Part model, mm, in its own coordinate system. A direction names the side the tool comes from. Round coordinates to 2 decimals unless told otherwise and drop trailing zeros. Loops run counter-clockwise (first coordinate to the right, second up) from the corner with the lowest first, then second, coordinate; pieces in that order, holes last. Notation, with made-up numbers: M 68.5,-22.75 L 111.5,-22.75 A16 ccw 111.5,-10.75 Z; hole C -9.75,32.25 d5. An arc over 180 degrees is marked long. Answer as CSV lines item,"result". Start each with the question number.
Item 1: Mould opens along X. For faces 1 (the cylindrical face through (-24, 51, 0)), 2 (the flat face through (-3, 22, -21)), 3 (the flat face through (-26, 19, 0)) say: pulls with the +X half, pulls with the -X half, needs draft (parallel to the pull), parting line crosses it, or undercut.
Item 2: Band-saw the part on B-B (z = -14.5). Count the separate pieces of the cut face and the enclosed holes in it, and give its area (3 significant figures).
Item 3: Band-saw the part on D-D (y = 47). Give the cut face in (x, z), and give its area (3 significant figures).
Item 4: Drop flat-ended pins along their axis: pin 1 Ø1.2 at (x, z) = (-25.5, 7.5) entering from -Y; pin 2 Ø6 at (x, z) = (-5, 11.5) entering from -Y. Give the stop position or say it passes through.
Item 5: Which spindle directions (+Z, -Z, +X, -X, +Y, -Y) get a long thin tool onto all of the face, cutting with end or side? Do faces 4 (the flat face through (-3, 37, -21)), 5 (the flat face through (-26, 58, 0)), 6 (the flat face through (-28, 53, 0)), 7 (the flat face through (-3, 55, 21)). Say none if no direction does.
Item 6: Wall check: line 1 (Z direction, x = 16.5, y = 57); line 2 (X direction, y = 18, z = 0); line 3 (Z direction, x = -16.5, y = 8.5). Give the ranges that are in metal, low to high.
Item 7: Band-saw the part on A-A (y = 56). Give the cut face in (x, z).
```python
from build123d import *

# Parameters (mm, degrees)
BOSS_EXTRUDE1_DEPTH     = 62
SKETCH2_R               = 18
BOSS_EXTRUDE2_DEPTH     = 2
SKETCH3_R               = 16
CUT_EXTRUDE1_DEPTH      = 65
CUT_EXTRUDE2_DEPTH      = 2
SKETCH6_R               = 3.5
CUT_EXTRUDE3_DEPTH      = 65
SKETCH7_W               = 48
SKETCH7_H               = 3
LPATTERN1_COUNT         = 9
LPATTERN1_PITCH         = 6
MIRROR1_COPY_1_SKETCH_W = 48
MIRROR1_COPY_1_SKETCH_H = 3
MIRROR1_COPY_2_SKETCH_W = 48
MIRROR1_COPY_2_SKETCH_H = 3
MIRROR1_COPY_3_SKETCH_W = 48
MIRROR1_COPY_3_SKETCH_H = 3
MIRROR1_COPY_4_SKETCH_W = 48
MIRROR1_COPY_4_SKETCH_H = 3
MIRROR1_COPY_5_SKETCH_W = 48
MIRROR1_COPY_5_SKETCH_H = 3
MIRROR1_COPY_6_SKETCH_W = 48
MIRROR1_COPY_6_SKETCH_H = 3
MIRROR1_COPY_7_SKETCH_W = 48
MIRROR1_COPY_7_SKETCH_H = 3
MIRROR1_COPY_8_SKETCH_W = 48
MIRROR1_COPY_8_SKETCH_H = 3
SKETCH9_W               = 48
SKETCH9_H               = 3
LPATTERN2_COUNT         = 9
LPATTERN2_PITCH         = 6


with BuildPart() as part:
    # Sketch1 → Boss-Extrude1 (new body)
    with BuildSketch(Plane(origin=(0, 0, 0), x_dir=(1, 0, 0), z_dir=(0, 1, 0))):
        with BuildLine():
            Line((-24, 22.5), (18, 22.5))
            ThreePointArc((18, 22.5), (20.828427125, 21.328427125), (22, 18.5))
            Line((22, 18.5), (22, -18.5))
            ThreePointArc((22, -18.5), (20.828427125, -21.328427125), (18, -22.5))
            Line((18, -22.5), (-24, -22.5))
            ThreePointArc((-24, -22.5), (-26.828427125, -21.328427125), (-28, -18.5))
            Line((-28, -18.5), (-28, 18.5))
            ThreePointArc((-28, 18.5), (-26.828427125, 21.328427125), (-24, 22.5))
        make_face()
    extrude(amount=BOSS_EXTRUDE1_DEPTH)

    # Sketch2 → Boss-Extrude2 (add)
    with BuildSketch(Plane.XZ):
        Circle(SKETCH2_R)
    extrude(amount=BOSS_EXTRUDE2_DEPTH)

    # Sketch3 → Cut-Extrude1 (cut, through all)
    with BuildSketch(Plane.XZ.offset(2)):
        Circle(SKETCH3_R)
    extrude(amount=-CUT_EXTRUDE1_DEPTH, mode=Mode.SUBTRACT)

    # Sketch5 → Cut-Extrude2 (cut)
    with BuildSketch(Plane(origin=(0, 62, 0), x_dir=(1, 0, 0), z_dir=(0, 1, 0))):
        with BuildLine():
            Line((-22.61, 2), (-11.427293838, 2))
            Line((-11.427293838, 2), (-11.427293838, -2))
            Line((-11.427293838, -2), (-22.61, -2))
            ThreePointArc((-22.61, -2), (-24.61, 0), (-22.61, 2))
        make_face()
    extrude(amount=-CUT_EXTRUDE2_DEPTH, mode=Mode.SUBTRACT)

    # Sketch6 → Cut-Extrude3 (cut, through all)
    with BuildSketch(Plane(origin=(0, 62, 0), x_dir=(1, 0, 0), z_dir=(0, 1, 0))):
        with Locations((16.263455967, 16.263455967)):
            Circle(SKETCH6_R)
        with Locations((16.263455967, -16.263455967)):
            Circle(SKETCH6_R)
        with Locations((-16.263455967, -16.263455967)):
            Circle(SKETCH6_R)
        with Locations((-16.263455967, 16.263455967)):
            Circle(SKETCH6_R)
    extrude(amount=-CUT_EXTRUDE3_DEPTH, mode=Mode.SUBTRACT)

    # Sketch7 → Cut-Revolve1 (revolve, cut)
    with BuildSketch(Plane(origin=(-3, 0, 0), x_dir=(0, 0, -1), z_dir=(1, 0, 0))):
        with Locations((-42.5, 56.5)):
            Rectangle(SKETCH7_W, SKETCH7_H)
    cut_revolve1 = revolve(axis=Axis((-3, 58, 66.5), (0, -1, 0)), mode=Mode.SUBTRACT)

    # LPattern1: Cut-Revolve1 ×9
    with Locations(*[(0, -i * LPATTERN1_PITCH, 0) for i in range(1, LPATTERN1_COUNT)]):
        add(cut_revolve1, mode=Mode.SUBTRACT)

    # Mirror1: Cut-Revolve1 across plane
    add(cut_revolve1.mirror(Plane.XY), mode=Mode.SUBTRACT)

    # Mirror1 copy 1 sketch → Mirror1 copy 1 (revolve, cut)
    with BuildSketch(Plane(origin=(-3, -6, 0), x_dir=(0, 0, 1), z_dir=(1, 0, 0))):
        with Locations((-42.5, -56.5)):
            Rectangle(MIRROR1_COPY_1_SKETCH_W, MIRROR1_COPY_1_SKETCH_H)
    revolve(axis=Axis((-3, 52, -66.5), (0, 1, 0)), mode=Mode.SUBTRACT)

    # Mirror1 copy 2 sketch → Mirror1 copy 2 (revolve, cut)
    with BuildSketch(Plane(origin=(-3, -12, 0), x_dir=(0, 0, 1), z_dir=(1, 0, 0))):
        with Locations((-42.5, -56.5)):
            Rectangle(MIRROR1_COPY_2_SKETCH_W, MIRROR1_COPY_2_SKETCH_H)
    revolve(axis=Axis((-3, 46, -66.5), (0, 1, 0)), mode=Mode.SUBTRACT)

    # Mirror1 copy 3 sketch → Mirror1 copy 3 (revolve, cut)
    with BuildSketch(Plane(origin=(-3, -18, 0), x_dir=(0, 0, 1), z_dir=(1, 0, 0))):
        with Locations((-42.5, -56.5)):
            Rectangle(MIRROR1_COPY_3_SKETCH_W, MIRROR1_COPY_3_SKETCH_H)
    revolve(axis=Axis((-3, 40, -66.5), (0, 1, 0)), mode=Mode.SUBTRACT)

    # Mirror1 copy 4 sketch → Mirror1 copy 4 (revolve, cut)
    with BuildSketch(Plane(origin=(-3, -24, 0), x_dir=(0, 0, 1), z_dir=(1, 0, 0))):
        with Locations((-42.5, -56.5)):
            Rectangle(MIRROR1_COPY_4_SKETCH_W, MIRROR1_COPY_4_SKETCH_H)
    revolve(axis=Axis((-3, 34, -66.5), (0, 1, 0)), mode=Mode.SUBTRACT)

    # Mirror1 copy 5 sketch → Mirror1 copy 5 (revolve, cut)
    with BuildSketch(Plane(origin=(-3, -30, 0), x_dir=(0, 0, 1), z_dir=(1, 0, 0))):
        with Locations((-42.5, -56.5)):
            Rectangle(MIRROR1_COPY_5_SKETCH_W, MIRROR1_COPY_5_SKETCH_H)
    revolve(axis=Axis((-3, 28, -66.5), (0, 1, 0)), mode=Mode.SUBTRACT)

    # Mirror1 copy 6 sketch → Mirror1 copy 6 (revolve, cut)
    with BuildSketch(Plane(origin=(-3, -36, 0), x_dir=(0, 0, 1), z_dir=(1, 0, 0))):
        with Locations((-42.5, -56.5)):
            Rectangle(MIRROR1_COPY_6_SKETCH_W, MIRROR1_COPY_6_SKETCH_H)
    revolve(axis=Axis((-3, 22, -66.5), (0, 1, 0)), mode=Mode.SUBTRACT)

    # Mirror1 copy 7 sketch → Mirror1 copy 7 (revolve, cut)
    with BuildSketch(Plane(origin=(-3, -42, 0), x_dir=(0, 0, 1), z_dir=(1, 0, 0))):
        with Locations((-42.5, -56.5)):
            Rectangle(MIRROR1_COPY_7_SKETCH_W, MIRROR1_COPY_7_SKETCH_H)
    revolve(axis=Axis((-3, 16, -66.5), (0, 1, 0)), mode=Mode.SUBTRACT)

    # Mirror1 copy 8 sketch → Mirror1 copy 8 (revolve, cut)
    with BuildSketch(Plane(origin=(-3, -48, 0), x_dir=(0, 0, 1), z_dir=(1, 0, 0))):
        with Locations((-42.5, -56.5)):
            Rectangle(MIRROR1_COPY_8_SKETCH_W, MIRROR1_COPY_8_SKETCH_H)
    revolve(axis=Axis((-3, 10, -66.5), (0, 1, 0)), mode=Mode.SUBTRACT)

    # Sketch9 → Cut-Revolve3 (revolve, cut)
    with BuildSketch(Plane.XY):
        with Locations((-48, 56.5)):
            Rectangle(SKETCH9_W, SKETCH9_H)
    cut_revolve3 = revolve(axis=Axis((-72, 58, 0), (0, -1, 0)), mode=Mode.SUBTRACT)

    # LPattern2: Cut-Revolve3 ×9
    with Locations(*[(0, -i * LPATTERN2_PITCH, 0) for i in range(1, LPATTERN2_COUNT)]):
        add(cut_revolve3, mode=Mode.SUBTRACT)


solid = part.part
```
Answer block:
1,face 1,"pulls with the -X half"
1,face 2,"undercut"
1,face 3,"needs draft"
2,separate pieces,"4"
2,enclosed holes,"0"
2,area,"1,480 mm^2"
3,outline,"M -28,-18.5 A4 ccw -24,-22.5 L 18,-22.5 A4 ccw 22,-18.5 L 22,18.5 A4 ccw 18,22.5 L -24,22.5 A4 ccw -28,18.5 Z; hole C -16.26,-16.26 d7; hole C -16.26,16.26 d7; hole C 0,0 d32; hole C 16.26,-16.26 d7; hole C 16.26,16.26 d7"
3,area,"1,280 mm^2"
4,pin 1,"stops at y = 0"
4,pin 2,"passes through"
5,face 4,"-Z"
5,face 5,"-X"
5,face 6,"+Z, -Z, -X, +Y, -Y"
5,face 7,"+Z"
6,line 1,"z = -22.5 to -19.76, -12.77 to 12.77, 19.76 to 22.5"
6,line 2,"x = -28 to -16, 16 to 22"
6,line 3,"z = -20.44 to -19.76, -12.77 to 12.77, 19.76 to 20.44"
7,outline,"M -27.96,-19.08 A4 ccw -24,-22.5 L -22.18,-22.5 A48 cw 16.18,-22.5 L 18,-22.5 A4 ccw 22,-18.5 L 22,18.5 A4 ccw 18,22.5 L 16.18,22.5 A48 cw -22.18,22.5 L -24,22.5 A4 ccw -27.96,19.08 A48 cw Z; hole C -16.26,-16.26 d7; hole C -16.26,16.26 d7; hole C 0,0 d32; hole C 16.26,-16.26 d7; hole C 16.26,16.26 d7"
